Verification items for the finished model (mm, model axes). Face numbers are marked on the shaded views. A direction names the side the tool comes from. Round coordinates to 2 decimals unless told otherwise and drop trailing zeros. Write each loop counter-clockwise with the first axis right and the second up, starting at its lowest first coordinate (ties: lowest second). Pieces come first, ordered by that corner, then holes. Notation, with made-up numbers: M 5,-17 L 59,-17 A31 ccw 59,21 Z; hole C 54,-15 d2. An arc over 180 degrees is marked long. One line per item, written item: value. Start each with the question number.
Item 1: Draft check along X on the marked faces 6, 7 and 8. Enter one of: +X half, -X half, draft (parallel to the pull), parting line (faces both ways), or undercut.
Item 2: Section check A-A, the plane x = -31.75. Record the cut outline in (y, z), then the cut area to 3 significant figures.
Item 3: Thickness scan on probe 1 along X at (y, z) = (2.5, 7.75) (3 decimals); probe 2 along X at (y, z) = (6, -2.75) (3 decimals); probe 3 along X at (y, z) = (6, -1.75) (3 decimals). Record the ranges inside material, lowest first. Write a range as from..to.
Item 4: Section check B-B, the plane x = 14.08. Record the cut outline in (y, z) (3 decimals).
Item 5: Section check C-C, the plane z = 10. Record the cut outline in (x, y) (3 decimals).
Item 6: Gauge pin test, flat ends, axial feed: pin 1 (0.9 mm diameter, centred on x = -17.5, y = -0.5, fed in from +Z); pin 2 (1.3 mm diameter, centred on y = 4.5, z = 1, fed in from -X); pin 3 (1.2 mm diameter, centred on x = 3, y = -1, fed in from +Z). Record the tip position at first contact, or that the pin passes through.
Item 7: Tool access check on the marked faces 1, 2, 3, 4 and 5. Record the directions out of +Z, -Z, +X, -X, +Y, -Y that give a thin tool (end or side, any length) a straight path to the whole face; none if there is none.
from build123d import *

# Parameters (mm, degrees)
SKETCH1_W                  = 69.85
SKETCH1_H                  = 25.4
SKETCH1_R                  = 1.5494
PCB_DEPTH                  = 1.6
TOP_FEATURES_W             = 17.9959
TOP_FEATURES_H             = 17.9959
GPS_ANTENNA_DEPTH          = 4.18
SKETCH2_3_W                = 4.74
SKETCH2_3_H                = 5.9817
JST_CONNECTOR_DEPTH        = 5.97
SKETCH2_4_W                = 6.35254
SKETCH2_4_H                = 15.64894
TERMINAL_BLOCK_DEPTH       = 8.63
BOTTOM_FEATURES_W          = 5.0038
BOTTOM_FEATURES_H          = 5.0038
CC1200_DEPTH               = 1.13
BOTTOM_FEATURES_4_W        = 12.6746
BOTTOM_FEATURES_4_H        = 10.5918
UBLOX_DEPTH                = 2.48
BOTTOM_FEATURES_5_W        = 8.636
BOTTOM_FEATURES_5_H        = 5.2705
FLASH_DEPTH                = 1.48
BOTTOM_FEATURES_6_W        = 5.04
BOTTOM_FEATURES_6_H        = 3.02
BARO_DEPTH                 = 1.22
BOTTOM_FEATURES_7_W        = 6.9723
BOTTOM_FEATURES_7_H        = 6.9723
UC_DEPTH                   = 0.87
BOTTOM_FEATURES_8_W        = 8.0391
BOTTOM_FEATURES_8_H        = 5.8293
USB_DEPTH                  = 2.57
BOTTOM_FEATURES_9_W        = 5.02666
BOTTOM_FEATURES_9_H        = 2.9972
ACCELEROMETER_DEPTH        = 1.12
TERMINALBLOCK_SOLDER_DEPTH = 2.17
TOP_FEATURES_5_R           = 5.885
BOSS_EXTRUDE13_DEPTH       = 6.53


with BuildPart() as part:
    # Sketch1 → PCB (new body)
    with BuildSketch(Plane(origin=(0, 0, 0), x_dir=(1, 0, 0), z_dir=(0, 1, 0))):
        Rectangle(SKETCH1_W, SKETCH1_H)
        with Locations(Location((-31.75, 9.525, 0), (0, 0, 270))):
            Circle(SKETCH1_R, mode=Mode.SUBTRACT)
        with Locations(Location((-31.75, -9.525, 0), (0, 0, 270))):
            Circle(SKETCH1_R, mode=Mode.SUBTRACT)
        with Locations(Location((25.4, 9.525, 0), (0, 0, 270))):
            Circle(SKETCH1_R, mode=Mode.SUBTRACT)
        with Locations(Location((25.4, -9.525, 0), (0, 0, 270))):
            Circle(SKETCH1_R, mode=Mode.SUBTRACT)
    extrude(amount=PCB_DEPTH)

    # top_features → gps_antenna (add)
    with BuildSketch(Plane(origin=(0, 1.6, 0), x_dir=(1, 0, 0), z_dir=(0, 1, 0))):
        with Locations((-3.15087, 0)):
            Rectangle(TOP_FEATURES_W, TOP_FEATURES_H)
    extrude(amount=GPS_ANTENNA_DEPTH)

    # Sketch2_3 → jst_connector (add)
    with BuildSketch(Plane(origin=(0, 1.6, 0), x_dir=(1, 0, 0), z_dir=(0, 1, 0))):
        with Locations((23.6044, 0)):
            Rectangle(SKETCH2_3_W, SKETCH2_3_H)
    extrude(amount=JST_CONNECTOR_DEPTH)

    # Sketch2_4 → terminal_block (add)
    with BuildSketch(Plane(origin=(0, 1.6, 0), x_dir=(1, 0, 0), z_dir=(0, 1, 0))):
        with Locations((31.74873, 0)):
            Rectangle(SKETCH2_4_W, SKETCH2_4_H)
    extrude(amount=TERMINAL_BLOCK_DEPTH)

    # bottom_features → cc1200 (add)
    with BuildSketch(Plane.XZ):
        with Locations((-18.6231, -2.0181)):
            Rectangle(BOTTOM_FEATURES_W, BOTTOM_FEATURES_H)
    extrude(amount=CC1200_DEPTH)

    # bottom_features_4 → ublox (add)
    with BuildSketch(Plane.XZ):
        with Locations((-9.4277, 6.2441)):
            Rectangle(BOTTOM_FEATURES_4_W, BOTTOM_FEATURES_4_H)
    extrude(amount=UBLOX_DEPTH)

    # bottom_features_5 → flash (add)
    with BuildSketch(Plane.XZ):
        with Locations((4.747, 9.22475)):
            Rectangle(BOTTOM_FEATURES_5_W, BOTTOM_FEATURES_5_H)
    extrude(amount=FLASH_DEPTH)

    # bottom_features_6 → baro (add)
    with BuildSketch(Plane.XZ):
        with Locations((13.695, 7.85)):
            Rectangle(BOTTOM_FEATURES_6_W, BOTTOM_FEATURES_6_H)
    extrude(amount=BARO_DEPTH)

    # bottom_features_7 → uC (add)
    with BuildSketch(Plane.XZ):
        with Locations((5.67885, -0.56385)):
            Rectangle(BOTTOM_FEATURES_7_W, BOTTOM_FEATURES_7_H)
    extrude(amount=UC_DEPTH)

    # bottom_features_8 → usb (add)
    with BuildSketch(Plane.XZ):
        with Locations((15.39545, -9.78535)):
            Rectangle(BOTTOM_FEATURES_8_W, BOTTOM_FEATURES_8_H)
    extrude(amount=USB_DEPTH)

    # bottom_features_9 → accelerometer (add)
    with BuildSketch(Plane.XZ):
        with Locations((-11.45833, -7.2514)):
            Rectangle(BOTTOM_FEATURES_9_W, BOTTOM_FEATURES_9_H)
    extrude(amount=ACCELEROMETER_DEPTH)

    # bottom_features_10 → terminalblock_solder (add)
    with BuildSketch(Plane.XZ):
        with BuildLine():
            Line((32.175, 6.4), (32.175, -6.4))
            ThreePointArc((32.175, -6.4), (31.315, -7.26), (30.455, -6.4))
            Line((30.455, -6.4), (30.455, 6.4))
            ThreePointArc((30.455, 6.4), (31.315, 7.26), (32.175, 6.4))
        make_face()
    extrude(amount=TERMINALBLOCK_SOLDER_DEPTH)

    # top_features_5 → Boss-Extrude13 (add)
    with BuildSketch(Plane(origin=(0, 1.6, 0), x_dir=(1, 0, 0), z_dir=(0, 1, 0))):
        with Locations(Location((14.08, 0, 0), (0, 0, 90))):
            Circle(TOP_FEATURES_5_R)
    extrude(amount=BOSS_EXTRUDE13_DEPTH)


solid = part.part
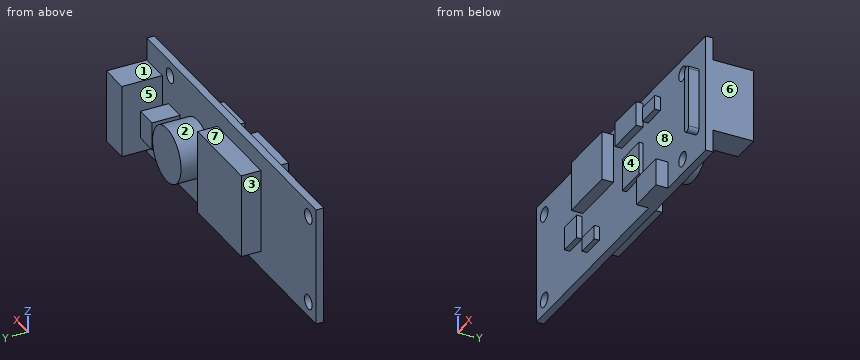
Response values:
1. face 6: +X half
1. face 7: draft
1. face 8: undercut
2. outline: M 0,-12.7 L 1.6,-12.7 L 1.6,-11.07 L 0,-11.07 Z; M 0,-7.98 L 1.6,-7.98 L 1.6,7.98 L 0,7.98 Z; M 0,11.07 L 1.6,11.07 L 1.6,12.7 L 0,12.7 Z
2. area: 30.7 mm2
3. probe 1: x = -12.149..5.847, 28.572..34.925
3. probe 2: x = 8.877..19.283, 21.234..25.974, 28.572..34.925
3. probe 3: x = 8.461..19.699, 21.234..25.974, 28.572..34.925
4. outline: M -2.57,-12.7 L 1.6,-12.7 L 1.6,-5.885 L 8.13,-5.885 L 8.13,5.885 L 1.6,5.885 L 1.6,12.7 L 0,12.7 L 0,9.36 L -1.22,9.36 L -1.22,6.34 L 0,6.34 L 0,-6.871 L -2.57,-6.871 Z
5. outline: M -34.925,0 L -33.225,0 L -33.225,1.6 L -34.925,1.6 Z; M -30.275,0 L -15.765,0 L -15.765,-2.48 L -3.09,-2.48 L -3.09,0 L 0.429,0 L 0.429,-1.48 L 9.065,-1.48 L 9.065,0 L 23.925,0 L 23.925,1.6 L -30.275,1.6 Z; M 26.875,0 L 34.925,0 L 34.925,1.6 L 26.875,1.6 Z
6. pin 1: stops at z = 0.48
6. pin 2: stops at x = -12.15
6. pin 3: stops at z = 11.86
7. face 1: +Z, +X, +Y
7. face 2: +Y
7. face 3: +Z, -Z, -X, +Y
7. face 4: -Z, -Y
7. face 5: +Z, -Z, +Y
